Geometry: final body of the model. Coordinates: model frame, mm. Coordinates: 2 decimals unless noted, no trailing zeros. Loops run counter-clockwise (first coordinate to the right, second up) from the corner with the lowest first, then second, coordinate; pieces in that order, holes last. Notation, with made-up numbers: (62.5, -36.5) -> (116.5, -36.5) arc R21 cw to (116.5, -0.5) -> close; hole circle Ø4 at (6.5, -39.5). An arc over 180 degrees is marked (long way). One line per item, written item: value. Start each with the question number.
Autodesk Inventor part; units mm, degrees
ref_plane "YZ Plane" through (0, 0, 0) normal (1, 0, 0) x (0, 1, 0)
ref_plane "XZ Plane" through (0, 0, 0) normal (0, 1, 0) x (-1, 0, 0)
ref_plane "XY Plane" through (0, 0, 0) normal (0, 0, 1) x (1, 0, 0)
sketch "スケッチ1" plane through (0, 0, 0) normal (0, 1, 0) x (-1, 0, 0)
  line L0 (25, 0) -> (-25, 0)
  line L1 (-25, 0) -> (-25, -159)
  line L2 (-25, -159) -> (25, -159)
  line L3 (25, -159) -> (25, 0)
  circle A0 centre (0, 0) radius 25
  circle A1 centre (0, 0) radius 57 construction
  circle A2 centre (0, -79.5) radius 22.5 construction
  circle A3 centre (0, 0) radius 75 construction
  circle A4 centre (0, -79.5) radius 10
  circle A5 centre (0, 0) radius 10
  circle A6 centre (0, -159) radius 10
  circle A7 centre (0, -159) radius 57 construction
  circle A8 centre (0, -159) radius 25
  circle A9 centre (0, -79.5) radius 27.5
  point P0 (25, -90.9564)
  point P1 (-25, -90.9564)
  dimension "d0" = 114
  dimension "d1" = 45
  dimension "d2" = 150
  dimension "d3" = 20
  dimension "d4" = 20
  dimension "d5" = 50
  dimension "d8" = 20
  dimension "d13" = 55
extrude "押し出し1" add sketch "スケッチ1" along normal blind 5.5 contours L3 A8 L1 A9 | A8 L2 A6 | L2 A6 A8
properties part number "ギアプレートupper_upper"
1. Line query: L1, parallel to X at y = 3.3, z = -159; L2, parallel to Z at x = 0, y = 1.45; L3, parallel to Z at x = 3.5, y = 3.75. Output: solid intervals per line, ascending. Write a range as [from, to].
2. Section D-D on x = -11. Return the cut outline in (y, z), plus the area to 3 significant figures.
3. Section B-B on z = -163.5. Return the cut outline in (x, y).
4. Pin query (flat end, axial travel): pin 1 Ø1 at (y, z) = (1, -167) entering from +X; pin 2 Ø1 at (x, y) = (2.5, 1.5) entering from +Z. Return the tip coordinate at first contact, or that it passes through.
5. Draft query along Z for faces 1 (the face through (2.17, 2.71, -149.24)), 2 (the face through (-0.55, 2.712, -183.994)), 3 (the face through (0, 3, -107)), 4 (the face through (25, 3, -125)). Return one class per face: released by +Z, released by -Z, zero draft, split by the parting line, or undercut.
6. Section A-A on x = 0. Return the cut outline in (y, z).
7. Section C-C on y = 0.85. Return the cut outline in (x, z), plus the area to 3 significant figures.
Checks:
1. L1: [-25, -10], [10, 25]
1. L2: [-184, -169], [-149, -107]
1. L3: [-183.75, -168.37], [-149.63, -106.78]
2. outline: (0, -181.45) -> (5.5, -181.45) -> (5.5, -104.7) -> (0, -104.7) -> close
2. area: 422 mm²
3. outline: (-24.59, 0) -> (-8.93, 0) -> (-8.93, 5.5) -> (-24.59, 5.5) -> close; (8.93, 0) -> (24.59, 0) -> (24.59, 5.5) -> (8.93, 5.5) -> close
4. pin 1: x = 23.85
4. pin 2: z = -106.84
5. face 1: undercut
5. face 2: released by -Z
5. face 3: released by +Z
5. face 4: zero draft
6. outline: (0, -184) -> (5.5, -184) -> (5.5, -169) -> (0, -169) -> close; (0, -149) -> (5.5, -149) -> (5.5, -107) -> (0, -107) -> close
7. outline: (-25, -159) arc R25 ccw to (25, -159) -> (25, -90.96) arc R27.5 cw to (-25, -90.96) -> close; hole circle Ø20 at (0, -159)
7. area: 3,490 mm²
